Input: dimensioned drawing with shaded views. Units: mm. Origin: part minimum x, y, z. Round coordinates to 2 decimals unless told otherwise and drop trailing zeros. Order: outer loops, then holes, each group sorted by start corner. A loop starts at its lowest first (then second) coordinate and runs counter-clockwise, first axis right, second up.
Item 1: Cut plane B-B on y = 31. Output: boundary loops of the cut face in (x, z), then the cut area to 4 significant figures.
Item 2: Cut plane C-C on z = 0.8. Output: boundary loops of the cut face in (x, y).
Item 3: Cut plane A-A on x = 11. Output: boundary loops of the cut face in (y, z).
Item 4: Line query: L1, parallel to Y at x = 51, z = 0.8; L2, parallel to Y at x = 14, z = 1.75; L3, parallel to X at y = 11.5, z = 2.1. Output: solid intervals per line, ascending.
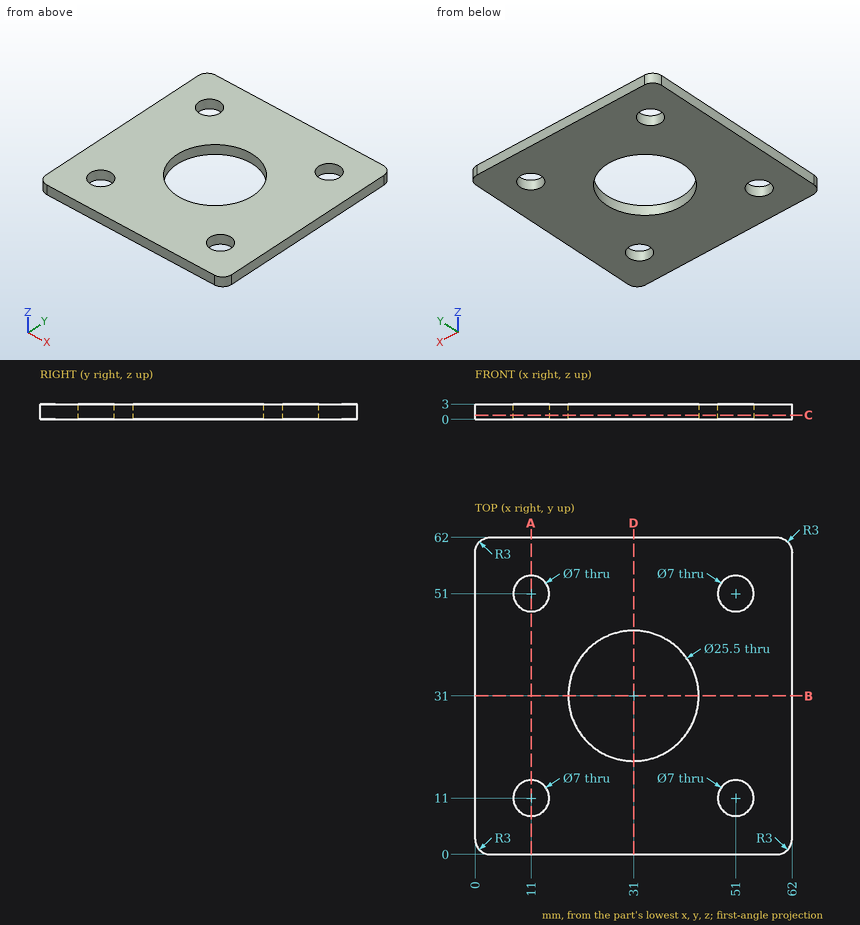
From the geometry:
1. outline: (0, 0) - (18.25, 0) - (18.25, 3) - (0, 3) - close; (43.75, 0) - (62, 0) - (62, 3) - (43.75, 3) - close
1. area: 109.5 mm2
2. outline: (0, 3) arc R3 ccw to (3, 0) - (59, 0) arc R3 ccw to (62, 3) - (62, 59) arc R3 ccw to (59, 62) - (3, 62) arc R3 ccw to (0, 59) - close; hole circle Ø7 at (11, 11); hole circle Ø7 at (11, 51); hole circle Ø25.5 at (31, 31); hole circle Ø7 at (51, 11); hole circle Ø7 at (51, 51)
3. outline: (0, 0) - (7.5, 0) - (7.5, 3) - (0, 3) - close; (14.5, 0) - (47.5, 0) - (47.5, 3) - (14.5, 3) - close; (54.5, 0) - (62, 0) - (62, 3) - (54.5, 3) - close
4. L1: y = 0 to 7.5, 14.5 to 47.5, 54.5 to 62
4. L2: y = 0 to 9.2, 12.8 to 49.2, 52.8 to 62
4. L3: x = 0 to 7.54, 14.46 to 47.54, 54.46 to 62
